Source: CAD feature listing. Evaluate the final solid. Frame: model axes, mm. A direction names the side the tool comes from. Give positions to 0.01 mm unless a question says otherwise; leave off trailing zeros. Loops run counter-clockwise (first coordinate to the right, second up) from the corner with the lowest first, then second, coordinate; pieces in that order, holes last. Notation, with made-up numbers: (87.5, 38.5) -> (112.5, 38.5) arc R37 ccw to (112.5, 77.5) -> close; hole circle Ø5 at (-18, 12.25). An arc over 180 degrees is marked (long way). Put each result on its own line as item: value.
```python
from build123d import *

# Parameters (mm, degrees)
F0_R     = 4.05
F0_R_2   = 6.075
F1_DEPTH = 15


with BuildPart() as f1:
    # F0 (on Front) → F1 (new body)
    with BuildSketch(Plane.XZ):
        with BuildLine():
            Line((20, 4.175), (29.708069, 4.175))
            ThreePointArc((29.708069, 4.175), (-30, 0), (29.708069, -4.175))
            Line((29.708069, -4.175), (20, -4.175))
            Line((20, -4.175), (20, 4.175))
        make_face()
        with Locations((-15.255275, -12.933545)):
            Circle(F0_R, mode=Mode.SUBTRACT)
        with Locations((12.933545, -15.255275)):
            Circle(F0_R, mode=Mode.SUBTRACT)
        with Locations((-12.933545, 15.255275)):
            Circle(F0_R, mode=Mode.SUBTRACT)
        Circle(F0_R_2, mode=Mode.SUBTRACT)
        with Locations((15.255275, 12.933545)):
            Circle(F0_R, mode=Mode.SUBTRACT)
    extrude(amount=F1_DEPTH)


solid = f1.part
```
(1) Reachability of faces 5 (the flat face through (20, -7, 0)), 6 (the flat face through (-0.6, -15, -6.2)) from +Z, -Z, +X, -X, +Y, -Y: full face, straight path, thin tool, end or side. Return the list, or none.
Calculated:
face 5: +X, +Y, -Y
face 6: +Z, -Z, +X, -X, -Y
(2) Section A-A on z = 0. Return loops of the section in (x, y) (3 decimals).
Calculated:
outline: (-30, -15) -> (-6.075, -15) -> (-6.075, 0) -> (-30, 0) -> close; (6.075, -15) -> (20, -15) -> (20, 0) -> (6.075, 0) -> close
(3) Line query: probe 1 along Z at (x, y) = (13.5, -3); probe 2 along X at (y, z) = (-11.5, 12); probe 3 along X at (y, z) = (-14, 16). Output: solid intervals per line, ascending. Write a range as from..to.
Calculated:
probe 1: z = -26.79..-19.27, -11.25..9.28, 16.58..26.79
probe 2: x = -27.5..-15.34, -10.52..11.31, 19.2..27.5
probe 3: x = -25.38..-16.91, -8.95..12.61, 17.9..25.38
(4) Section C-C on y = -5. Return loops of the section in (x, z) (3 decimals).
Calculated:
outline: (20, -4.175) -> (20, 4.175) -> (29.708, 4.175) arc R30 ccw (long way) to (29.708, -4.175) -> close; hole circle Ø8.1 at (-15.255, -12.934); hole circle Ø8.1 at (-12.934, 15.255); hole circle Ø12.15 at (0, 0); hole circle Ø8.1 at (12.934, -15.255); hole circle Ø8.1 at (15.255, 12.934)
(5) Draft query along Z for faces 1 (the cylindrical face through (12.04, -7.4, 10.47)), 2 (the cylindrical face through (-29.974, -7.395, 1.26)), 3 (the cylindrical face through (14.8, -7.4, -18.85)), 4 (the flat face through (-0.6, 0, -6.2)). Return one class per face: released by +Z, released by -Z, zero draft, split by the parting line, or undercut.
Calculated:
face 1: undercut
face 2: split by the parting line
face 3: undercut
face 4: zero draft
(6) First-contact query: P1, Ø2, axis at y = -2.5, z = 8.5, coming from the -X side; P2, Ø5, axis at x = 12.93, z = -15.26, coming from the -Y side; P3, Ø5, axis at x = 24, y = -9, coming from the +Z side; P4, Ø1, axis at x = -18.5, y = -6.5, coming from the +Z side. Flat tips, straight axial feed; report the tip coordinate or a pass-through.
Calculated:
P1: stops at x = -29.05
P2: passes through
P3: stops at z = 20.92
P4: stops at z = 24
(7) Section B-B on x = 0. Return loops of the section in (y, z) (3 decimals).
Calculated:
outline: (-15, -30) -> (0, -30) -> (0, -6.075) -> (-15, -6.075) -> close; (-15, 6.075) -> (0, 6.075) -> (0, 30) -> (-15, 30) -> close
